from build123d import *

# Parameters (mm, degrees)
SKETCH1_W         = 5.5
SKETCH1_H         = 6
SKETCH1_H_2       = 2.5
CIRPATTERN1_COUNT = 8
FILLET1_R         = 1.5
FILLET2_R         = 0.5


with BuildPart() as part:
    # Sketch1 → Revolve1 (revolve)
    with BuildSketch(Plane.XY, mode=Mode.PRIVATE) as revolve1_sk:
        with Locations((2.75, -3)):
            Rectangle(SKETCH1_W, SKETCH1_H)
        Polygon((1.5, -6), (0, -6), (0, -8), align=None)
        with Locations((2.75, 1.25)):
            Rectangle(SKETCH1_W, SKETCH1_H_2)
    revolve(revolve1_sk.sketch.rotate(Axis((-1000, -44.5, 0), (1, 0, 0)), 90), axis=Axis((-1000, -44.5, 0), (1, 0, 0)))

    # Sketch6 → M3 Clearance Hole3 (revolve, cut)
    with BuildSketch(Plane(origin=(5.5, -76.100440255, 26.900969791), x_dir=(0, 0, -1), z_dir=(0, 1, 0))):
        Polygon((0, 0), (0, 6.581549114), (1.8, 5.5), (1.8, 0), align=None)
    m3_clearance_hole3 = revolve(axis=Axis((11.85, -76.100440255, 26.900969791), (-1, 0, 0)), mode=Mode.SUBTRACT)

    # CirPattern1: M3 Clearance Hole3 ×8 about axis
    cirpattern1_axis = Axis((0, -44.5, 0), (1, 0, 0))
    for i in range(1, CIRPATTERN1_COUNT):
        add(m3_clearance_hole3.rotate(cirpattern1_axis, i * 360 / CIRPATTERN1_COUNT), mode=Mode.SUBTRACT)

    # Fillet1
    fillet1_edges = [part.edges().sort_by_distance(p)[0] for p in [
        (5.5, -44.5, -47),
    ]]
    fillet(fillet1_edges, radius=FILLET1_R)

    # Fillet2
    fillet2_edges = [part.edges().sort_by_distance(p)[0] for p in [
        (0, -44.5, -47),
    ]]
    fillet(fillet2_edges, radius=FILLET2_R)


solid = part.part
Design review of the part built by this model. Coordinates are the model's own, in mm. A direction names the side the tool comes from. Round coordinates to 2 decimals unless told otherwise and drop trailing zeros. Order: outer loops, then holes, each group sorted by start corner. A loop starts at its lowest first (then second) coordinate and runs counter-clockwise, first axis right, second up.
1) Machinability: for faces 1 (the cylindrical face through (3.53, -21.07, -30.55)), 2 (the cylindrical face through (2.8, -12.8, -28.7)), which of the approach directions +Z, -Z, +X, -X, +Y, -Y give a long, thin tool a straight path to every point of the face, cutting with its end or side? Answer none if there is none.
The answers:
face 1: +X
face 2: +X, -X
2) Clearance check with flat-ended pins moving along their axes: pin 1 Ø6 at (y, z) = (-76.1, 26.9) entering from +X; pin 2 Ø1 at (x, y) = (5, -76.5) entering from -Z; pin 3 Ø3 at (y, z) = (-47.82, 41.37) entering from +X; pin 4 Ø1.5 at (x, z) = (3, 31) entering from -Y. State where each tip first meets the part, or that it passes through.
The answers:
pin 1: stops at x = 5.5
pin 2: stops at z = -34.56
pin 3: passes through
pin 4: stops at y = -80.47
3) For L1, parallel to Y at x = 1.45, z = -26; L2, parallel to Y at x = 2.3, z = -26.5; L3, parallel to Z at x = 0.5, y = -13.5, list the stretches that pass through material, from the lowest coordinate up.
The answers:
L1: y = -83.65 to -72.8, -16.2 to -14.46, -11.34 to -5.35
L2: y = -83.32 to -72.43, -16.57 to -14.65, -11.14 to -5.68
L3: z = -35.33 to -28.6, -25.2 to -20.5, 20.5 to 35.33
4) Draft analysis for pull direction Z (two halves, no side actions). For faces 3 (the cylindrical face through (2.788, -16.171, 30.505)), 4 (the cylindrical face through (2.788, -69.684, -32.141)), 5 (the cylindrical face through (2.274, -2.803, 21.688)), 6 (the flat face through (0, -13.7, 20.4)), state which applies: released by +Z, released by -Z, zero draft, split by the parting line, or undercut.
The answers:
face 3: undercut
face 4: undercut
face 5: split by the parting line
face 6: zero draft
5) Consider section B-B (z = 0). State the section outline as (x, y) points.
The answers:
outline: (0, -91) arc R0.5 ccw to (0.5, -91.5) - (4, -91.5) arc R1.5 ccw to (5.5, -90) - (5.5, -83) - (1.5, -83) - (0, -81) - close; (0, -8) - (1.5, -6) - (5.5, -6) - (5.5, 1) arc R1.5 ccw to (4, 2.5) - (0.5, 2.5) arc R0.5 ccw to (0, 2) - close
6) Consider section A-A (y = -44.5). State the section outline as (x, z) points.
The answers:
outline: (0, -46.5) arc R0.5 ccw to (0.5, -47) - (4, -47) arc R1.5 ccw to (5.5, -45.5) - (5.5, -38.5) - (1.5, -38.5) - (0, -36.5) - close; (0, 36.5) - (1.5, 38.5) - (5.5, 38.5) - (5.5, 45.5) arc R1.5 ccw to (4, 47) - (0.5, 47) arc R0.5 ccw to (0, 46.5) - close
7) Consider section C-C (x = 2.7). Count the separate pieces of the cut face and the enclosed holes in it, plus the area to 3 significant figures.
The answers:
separate pieces: 1
enclosed holes: 9
area: 2,200 mm2
